Geometry: final body of the model. Coordinates: model frame, mm. Face numbers are marked on the shaded views. A direction names the side the tool comes from. Give positions to 0.01 mm unless a question says otherwise; leave off trailing zeros. Loops run counter-clockwise (first coordinate to the right, second up) from the corner with the lowest first, then second, coordinate; pieces in that order, holes last. Notation, with made-up numbers: (38.25, 49.5) - (97.25, 49.5) arc R17 cw to (97.25, 56.5) - close; hole circle Ø6 at (86.25, 70). An arc over 180 degrees is marked (long way). Use one line per item in the form item = value.
```python
from build123d import *

# Parameters (mm, degrees)
SKETCH_1_W          = 32
SKETCH_1_H          = 10
EXTRUDE_1_DEPTH     = 5
SKETCH_2_R          = 2.1
CUT_EXTRUDE_1_DEPTH = 11
EXTRUDE_2_DEPTH     = 4
SKETCH_5_R          = 1.1
CUT_EXTRUDE_2_DEPTH = 6
CUT_EXTRUDE_3_DEPTH = 1.6


with BuildPart() as part:
    # Эскиз1 → Бобышка-Вытянуть1 (new body)
    with BuildSketch(Plane.XY):
        with Locations((16, 5)):
            Rectangle(SKETCH_1_W, SKETCH_1_H)
    extrude(amount=EXTRUDE_1_DEPTH)

    # Эскиз2 → Вырез-Вытянуть1 (cut, through all)
    with BuildSketch(Plane(origin=(0, 10, 0), x_dir=(1, 0, 0), z_dir=(0, 1, 0))):
        with Locations((8.575, -5.5)):
            Circle(SKETCH_2_R)
        with Locations((23.425, -5.5)):
            Circle(SKETCH_2_R)
    extrude(amount=-CUT_EXTRUDE_1_DEPTH, mode=Mode.SUBTRACT)

    # Эскиз4 → Бобышка-Вытянуть2 (add)
    with BuildSketch(Plane.XZ.offset(-6)):
        with BuildLine():
            Line((6.535392195, 5), (7.055131585, 5))
            ThreePointArc((7.055131585, 5), (8.575, 3.9), (10.094868415, 5))
            Line((10.094868415, 5), (10.614607805, 5))
            ThreePointArc((10.614607805, 5), (8.575, 3.4), (6.535392195, 5))
        make_face()
        with BuildLine():
            Line((21.385392195, 5), (21.905131585, 5))
            ThreePointArc((21.905131585, 5), (23.425, 3.9), (24.944868415, 5))
            Line((24.944868415, 5), (25.464607805, 5))
            ThreePointArc((25.464607805, 5), (23.425, 3.4), (21.385392195, 5))
        make_face()
    extrude(amount=EXTRUDE_2_DEPTH)

    # Эскиз5 → Вырез-Вытянуть2 (cut, through all)
    with BuildSketch(Plane(origin=(0, 0, 0), x_dir=(-1, 0, 0), z_dir=(0, 0, -1))):
        with Locations((-3.5, 5)):
            Circle(SKETCH_5_R)
        with Locations((-16, 5)):
            Circle(SKETCH_5_R)
        with Locations((-28.5, 5)):
            Circle(SKETCH_5_R)
    extrude(amount=-CUT_EXTRUDE_2_DEPTH, mode=Mode.SUBTRACT)

    # Эскиз6 → Вырез-Вытянуть3 (cut)
    with BuildSketch(Plane(origin=(0, 0, 0), x_dir=(-1, 0, 0), z_dir=(0, 0, -1))):
        Polygon((-16, 2.575128869), (-13.9, 3.787564435), (-13.9, 6.212435565), (-16, 7.424871131), (-18.1, 6.212435565), (-18.1, 3.787564435), align=None)
        Polygon((-3.5, 2.575128869), (-1.4, 3.787564435), (-1.4, 6.212435565), (-3.5, 7.424871131), (-5.6, 6.212435565), (-5.6, 3.787564435), align=None)
        Polygon((-28.5, 2.575128869), (-26.4, 3.787564435), (-26.4, 6.212435565), (-28.5, 7.424871131), (-30.6, 6.212435565), (-30.6, 3.787564435), align=None)
    extrude(amount=-CUT_EXTRUDE_3_DEPTH, mode=Mode.SUBTRACT)


solid = part.part
```
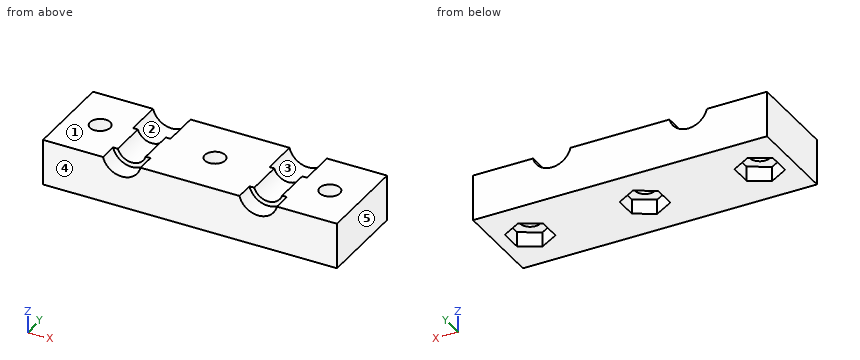
(1) Cut plane B-B (z = 1.25). Return the cut outline in (x, y).
Solution:
outline = (0, 0) - (32, 0) - (32, 10) - (0, 10) - close; hole (1.4, 3.79) - (3.5, 2.58) - (5.6, 3.79) - (5.6, 6.21) - (3.5, 7.42) - (1.4, 6.21) - close; hole (13.9, 3.79) - (16, 2.58) - (18.1, 3.79) - (18.1, 6.21) - (16, 7.42) - (13.9, 6.21) - close; hole (26.4, 3.79) - (28.5, 2.58) - (30.6, 3.79) - (30.6, 6.21) - (28.5, 7.42) - (26.4, 6.21) - close
(2) Access query for the marked faces 1 and 2. Directions: +Z, -Z, +X, -X, +Y, -Y. A direction counts if a zero-diameter tool reaches every point of the face in a straight line with its end or side. Return the directions, or none.
Solution:
face_1 = +Z, +X, -X, +Y, -Y
face_2 = +Z, +Y
(3) Pull-direction query (X, two-part tool) for the marked faces 3, 4 and 5; classes: released by +X, released by -X, zero draft, split by the parting line, or undercut.
Solution:
face_3 = undercut
face_4 = zero draft
face_5 = released by +X
(4) Material intervals for L1, parallel to X at y = 3.5, z = 0.95; L2, parallel to Y at x = 16, z = 3.8; L3, parallel to X at y = 7, z = 0.9, sorted ascending. Write a range as from..to.
Solution:
L1 = 0..1.9, 5.1..14.4, 17.6..26.9, 30.1..32
L2 = 0..3.9, 6.1..10
L3 = 0..2.76, 4.24..15.26, 16.74..27.76, 29.24..32
(5) Cut plane A-A (y = 5). Give the number of separate pieces and of enclosed holes in the cut face, plus the area to 3 significant figures.
Solution:
separate_pieces = 4
enclosed_holes = 0
area = 113 mm2
(6) Pin query (flat end, axial travel): P1, Ø2, axis at x = 3.5, y = 5, coming from the +Z side; P2, Ø2, axis at x = 16, y = 5.5, coming from the -Z side; P3, Ø0.5, axis at x = 23.5, z = 4, coming from the -Y side. Return the tip coordinate at first contact, or that it passes through.
Solution:
P1 = through
P2 = 1.6
P3 = 2
(7) Cut plane C-C (y = 8). Return the cut outline in (x, z) (3 decimals), plus the area to 3 significant figures.
Solution:
outline = (0, 0) - (32, 0) - (32, 5) - (25.465, 5) arc R2.1 cw to (21.385, 5) - (10.615, 5) arc R2.1 cw to (6.535, 5) - (0, 5) - close
area = 150 mm2
(8) Cut plane D-D (y = 6.75). Return the cut outline in (x, z) (3 decimals), plus the area to 3 significant figures.
Solution:
outline = (0, 0) - (2.331, 0) - (2.331, 1.6) - (4.669, 1.6) - (4.669, 0) - (14.831, 0) - (14.831, 1.6) - (17.169, 1.6) - (17.169, 0) - (27.331, 0) - (27.331, 1.6) - (29.669, 1.6) - (29.669, 0) - (32, 0) - (32, 5) - (25.465, 5) arc R2.1 cw to (21.385, 5) - (10.615, 5) arc R2.1 cw to (6.535, 5) - (0, 5) - close
area = 139 mm2
